```python
from build123d import *

# Parameters (mm, degrees)
SKETCH1_R           = 1.439670622
SKETCH1_R_2         = 1.5
SKETCH1_W           = 20
SKETCH1_H           = 2
BOSS_EXTRUDE3_DEPTH = 1.2
BOSS_EXTRUDE4_DEPTH = 2.2


with BuildPart() as part:
    # Sketch1 → Boss-Extrude3 (new body)
    # profile 1 of 3: a face of its own
    with BuildSketch(Plane(origin=(0, 0, 0), x_dir=(1, 0, 0), z_dir=(0, 1, 0))):
        Polygon((34.5, 0), (29, 0), (29, -6), (35, -6), (35, 0), align=None)
        with Locations(Location((32, -3, 0), (0, 0, 270))):
            Circle(SKETCH1_R, mode=Mode.SUBTRACT)
    # profile 2 of 3: a face of its own
    with BuildSketch(Plane(origin=(0, 0, 0), x_dir=(1, 0, 0), z_dir=(0, 1, 0))):
        Polygon((0, 29.5), (0, 0), (0.5, 0), (0.5, 22.5), (34.5, 22.5), (34.5, 0), (35, 0), (35, 29.5), align=None)
        with Locations(Location((3, 26.5, 0), (0, 0, 270))):
            Circle(SKETCH1_R_2, mode=Mode.SUBTRACT)
        with Locations((17.5, 26)):
            Rectangle(SKETCH1_W, SKETCH1_H, mode=Mode.SUBTRACT)
        with Locations(Location((32, 26.5, 0), (0, 0, 270))):
            Circle(SKETCH1_R_2, mode=Mode.SUBTRACT)
    # profile 3 of 3: a face of its own
    with BuildSketch(Plane(origin=(0, 0, 0), x_dir=(1, 0, 0), z_dir=(0, 1, 0))):
        Polygon((0.5, 0), (0, 0), (0, -6), (6, -6), (6, 0), align=None)
        with Locations(Location((3, -3, 0), (0, 0, 270))):
            Circle(SKETCH1_R_2, mode=Mode.SUBTRACT)
    extrude(amount=BOSS_EXTRUDE3_DEPTH)

    # Sketch1_7 → Boss-Extrude4 (add)
    with BuildSketch(Plane(origin=(0, 0, 0), x_dir=(1, 0, 0), z_dir=(0, 1, 0))):
        Polygon((0.5, 22.5), (0.5, 0), (6, 0), (29, 0), (34.5, 0), (34.5, 22.5), align=None)
    extrude(amount=BOSS_EXTRUDE4_DEPTH)


solid = part.part
```
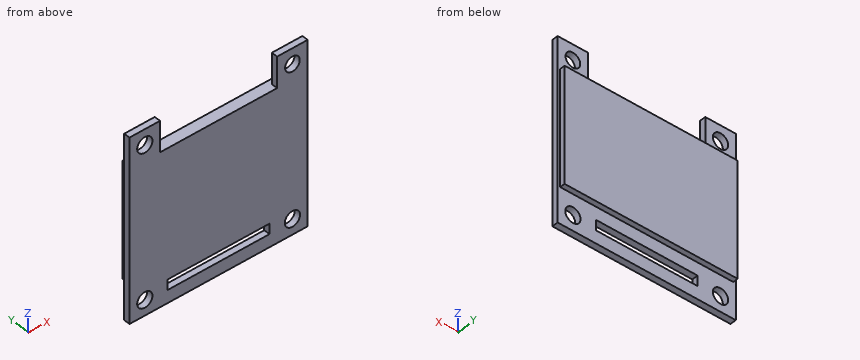
Read the model definition and answer for the solid it produces. Units are mm, in the model's axes. Coordinates: 2 decimals unless noted, no trailing zeros. Loops run counter-clockwise (first coordinate to the right, second up) from the corner with the lowest first, then second, coordinate; pieces in that order, holes last.
(1) Consider line 1 along X through (y, z) = (0.5, 3); line 2 along X through (y, z) = (0.75, -26.5); line 3 along Z through (x, y) = (8.5, 0.4). Determine where each line is inside the solid, lowest interval first.
Solution:
line 1: x = 0 to 1.5, 4.5 to 6, 29 to 30.56, 33.44 to 35
line 2: x = 0 to 1.5, 4.5 to 7.5, 27.5 to 30.5, 33.5 to 35
line 3: z = -29.5 to -27, -25 to 0
(2) The part is cut by section B-B (z = 3). Determine the outline of the cut face in (x, y).
Solution:
outline: (0, 0) - (1.5, 0) - (1.5, 1.2) - (0, 1.2) - close; (4.5, 0) - (6, 0) - (6, 1.2) - (4.5, 1.2) - close; (29, 0) - (30.56, 0) - (30.56, 1.2) - (29, 1.2) - close; (33.44, 0) - (35, 0) - (35, 1.2) - (33.44, 1.2) - close
(3) The part is cut by section C-C (y = 0.75). Determine the outline of the cut face in (x, z), and give its area (3 significant figures).
Solution:
outline: (0, -29.5) - (35, -29.5) - (35, 6) - (29, 6) - (29, 0) - (6, 0) - (6, 6) - (0, 6) - close; hole circle Ø3 at (3, -26.5); hole circle Ø3 at (3, 3); hole (7.5, -27) - (27.5, -27) - (27.5, -25) - (7.5, -25) - close; hole circle Ø3 at (32, -26.5); hole circle Ø2.88 at (32, 3)
area: 1,040 mm2
(4) The part is cut by section D-D (x = 3). Determine the outline of the cut face in (y, z), and give its area (3 significant figures).
Solution:
outline: (0, -29.5) - (1.2, -29.5) - (1.2, -28) - (0, -28) - close; (0, -25) - (1.2, -25) - (1.2, -22.5) - (2.2, -22.5) - (2.2, 0) - (1.2, 0) - (1.2, 1.5) - (0, 1.5) - close; (0, 4.5) - (1.2, 4.5) - (1.2, 6) - (0, 6) - close
area: 57.9 mm2
(5) The part is cut by section A-A (x = 32). Determine the outline of the cut face in (y, z), and give its area (3 significant figures).
Solution:
outline: (0, -29.5) - (1.2, -29.5) - (1.2, -28) - (0, -28) - close; (0, -25) - (1.2, -25) - (1.2, -22.5) - (2.2, -22.5) - (2.2, 0) - (1.2, 0) - (1.2, 1.56) - (0, 1.56) - close; (0, 4.44) - (1.2, 4.44) - (1.2, 6) - (0, 6) - close
area: 58.0 mm2
(6) Flat-ended cylindrical pins translate along their axes: pin 1 Ø1.8 at (x, z) = (3, 3) entering from +Y; pin 2 Ø1 at (x, y) = (9.5, 0.5) entering from +Z; pin 3 Ø1.1 at (y, z) = (2, -12) entering from +X; pin 4 Ø1.1 at (y, z) = (2, -5.5) entering from -X. Find the tip coordinate at first contact, or state that the pin passes through.
Solution:
pin 1: passes through
pin 2: stops at z = 0
pin 3: stops at x = 34.5
pin 4: stops at x = 0.5
